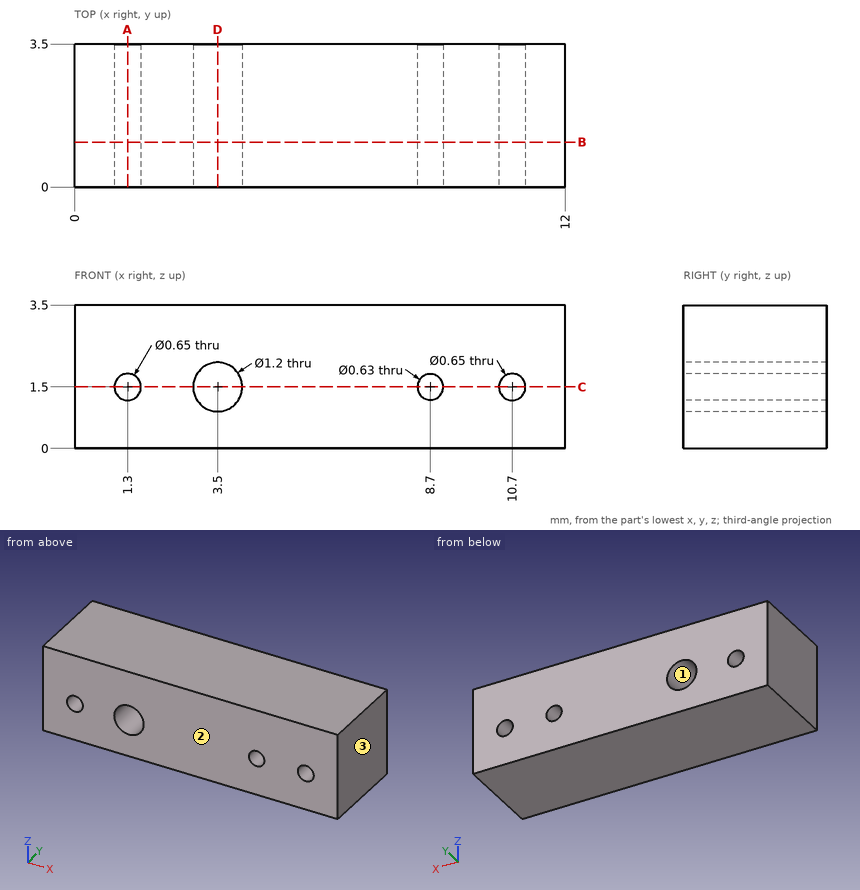
Drawing for the job (mm, zero at the part's lowest x, y, z). Coordinates: 2 decimals unless noted, no trailing zeros. Order: outer loops, then holes, each group sorted by start corner. A loop starts at its lowest first (then second) coordinate and runs counter-clockwise, first axis right, second up. Notation, with made-up numbers: (-3.5, 24) -> (5.5, 24) arc R15 ccw to (5.5, 47) -> close; hole circle Ø6 at (61, -28.75). An arc over 180 degrees is marked (long way). One line per item, written item: value.
(1) Mould opens along X. For the marked faces 1, 2 and 3 say: pulls with the +X half, pulls with the -X half, needs draft (parallel to the pull), parting line crosses it, or undercut.
Checked values:
face 1: undercut
face 2: needs draft
face 3: pulls with the +X half
(2) Slice it at A-A, the plane x = 1.3. List the corners of the cut face in (y, z) (3 decimals).
Checked values:
outline: (0, 0) -> (3.5, 0) -> (3.5, 1.175) -> (0, 1.175) -> close; (0, 1.825) -> (3.5, 1.825) -> (3.5, 3.5) -> (0, 3.5) -> close
(3) Drop a flat-ended pin along its axis: pin 1 Ø1 at (x, z) = (3.5, 1.5) entering from -Y. Give the stop position or say it passes through.
Checked values:
pin 1: through
(4) Slice it at B-B, the plane y = 1.1. List the corners of the cut face in (x, z) (3 decimals), plus the area to 3 significant figures.
Checked values:
outline: (0, 0) -> (12, 0) -> (12, 3.5) -> (0, 3.5) -> close; hole circle Ø0.65 at (1.3, 1.5); hole circle Ø1.2 at (3.5, 1.5); hole circle Ø0.63 at (8.7, 1.5); hole circle Ø0.65 at (10.7, 1.5)
area: 39.9 mm2
(5) Slice it at C-C, the plane z = 1.5. List the corners of the cut face in (x, y) (3 decimals), plus the area to 3 significant figures.
Checked values:
outline: (0, 0) -> (0.975, 0) -> (0.975, 3.5) -> (0, 3.5) -> close; (1.625, 0) -> (2.9, 0) -> (2.9, 3.5) -> (1.625, 3.5) -> close; (4.1, 0) -> (8.385, 0) -> (8.385, 3.5) -> (4.1, 3.5) -> close; (9.015, 0) -> (10.375, 0) -> (10.375, 3.5) -> (9.015, 3.5) -> close; (11.025, 0) -> (12, 0) -> (12, 3.5) -> (11.025, 3.5) -> close
area: 31.0 mm2
(6) Probe line 1 (X direction, y = 1.6, z = 1.5) (3 decimals); line 2 (Z direction, x = 10.7, y = 1.3) (3 decimals); line 3 (Z direction, x = 3.5, y = 2.2). List the from-to ranges inside material, lowest first. Write a range as [from, to].
Checked values:
line 1: [0, 0.975], [1.625, 2.9], [4.1, 8.385], [9.015, 10.375], [11.025, 12]
line 2: [0, 1.175], [1.825, 3.5]
line 3: [0, 0.9], [2.1, 3.5]
(7) Slice it at D-D, the plane x = 3.5. List the corners of the cut face in (y, z), plus the area to 3 significant figures.
Checked values:
outline: (0, 0) -> (3.5, 0) -> (3.5, 0.9) -> (0, 0.9) -> close; (0, 2.1) -> (3.5, 2.1) -> (3.5, 3.5) -> (0, 3.5) -> close
area: 8.05 mm2
